Geometry check sheet. Reference: the model listing, model coordinates, mm. A direction names the side the tool comes from. Give positions to 0.01 mm unless a question says otherwise; leave off trailing zeros. Loops run counter-clockwise (first coordinate to the right, second up) from the corner with the lowest first, then second, coordinate; pieces in that order, holes last. Notation, with made-up numbers: (-33, 10) - (16, 10) arc R21 ccw to (16, 38) - close; hole circle Ø1 at (15.25, -1.5). An arc over 180 degrees is marked (long way). Write item = value, one per line. Start each with the question number.
Autodesk Inventor part; units mm, degrees
ref_plane "YZ Plane" through (0, 0, 0) normal (1, 0, 0) x (0, 1, 0)
ref_plane "XZ Plane" through (0, 0, 0) normal (0, 1, 0) x (-1, 0, 0)
ref_plane "XY Plane" through (0, 0, 0) normal (0, 0, 1) x (1, 0, 0)
sketch "Sketch1" plane through (0, 0, 0) normal (0, 0, 1) x (1, 0, 0)
  line L0 (0, 0) -> (114.3, 0)
  line L1 (114.3, 0) -> (114.3, 25.4)
  line L2 (114.3, 25.4) -> (0, 25.4)
  line L3 (0, 25.4) -> (0, 0)
  dimension "d0" = 114.3
  dimension "d1" = 25.4
extrude "Plate1" add sketch "Sketch1" along normal blind 3.048
sketch "Sketch2" plane through (114.3, 22.352, 3.048) normal (0, 1, 0) x (-1, 0, 0)
  line L0 (114.3, 0) -> (0, 0)
  line L1 (0, 0) -> (0, -25.4)
  line L2 (0, -25.4) -> (114.3, -25.4)
  line L3 (114.3, -25.4) -> (114.3, 0)
edge flange "Flange1" height 25.4 angle 90 thickness 3.048 bend radius 3.048 thickness toward (0, 1, 0) relief tear relief width 3.048 relief depth 1.524 edges at (57.15, 25.4, 0) wall of the first edge with corners at (0, 22.352, 3.048) (114.3, 22.352, 3.048) (114.3, 22.352, -22.352) (0, 22.352, -22.352)
bend "Bend1"
corner "Corner1"
hole "Hole1" at (101.6, 9.652, 0) direction (0, 0, 1) diameter 6.35 end through all
hole "Hole2" at (25.4, 9.652, 0) direction (0, 0, 1) diameter 6.35 end through all
equation "\"d20\" = Thickness"
equation "\"d29\" = Thickness"
equation "\"d3\" = BendReliefWidth"
equation "\"d4\" = BendReliefDepth"
equation "\"d5\" = MinimumRemnant"
equation "\"d6\" = BendRadius"
equation "\"d9\" = BendRadius"
equation "\"d10\" = CornerReliefSize"
equation "\"d11\" = GapSize"
equation "\"d12\" = JacobiRadiusSize"
equation "\"BendRadius\" = Thickness"
equation "\"BendReliefWidth\" = Thickness"
equation "\"BendReliefDepth\" = 0.5 * Thickness"
equation "\"CornerReliefSize\" = 4 * Thickness"
equation "\"MinimumRemnant\" = 2 * Thickness"
equation "\"TransitionRadius\" = BendRadius"
equation "\"JacobiRadiusSize\" = BendRadius"
equation "\"GapSize\" = Thickness"
equation "\"d2\" = BendRadius"
properties part number "Chain Tension - L Bracket"
1) Cross-section at D-D on z = -1.5. Enter the section's corners in (x, y).
2) Tool access check on faces 4 (the face through (56, 10, 0)), 5 (the face through (58, 25.4, -13)). Record the directions out of +Z, -Z, +X, -X, +Y, -Y that give a thin tool (end or side, any length) a straight path to the whole face; none if there is none.
3) Cross-section at B-B on y = 10.5. Enter the section's corners in (x, z), and give its area (3 significant figures).
4) Material ranges on line 1 along Z through (x, y) = (109, 4.5); line 2 along Y through (x, z) = (98.5, -18.75); line 3 along Y through (x, z) = (25.4, 1), recorded low to high.
5) Cross-section at C-C on z = -15.5. Enter the section's corners in (x, y).
6) Cross-section at A-A on x = 25.4. Enter the section's corners in (y, z), and give its area (3 significant figures).
7) Gauge pin test, flat ends, axial feed: P1, Ø1, axis at x = 66, y = 8, coming from the -Z side; P2, Ø4, axis at x = 24.5, z = -12.5, coming from the -Y side; P3, Ø4, axis at x = 74.5, y = 22, coming from the +Z side; P4, Ø1.5, axis at y = 11.5, z = -2.5, coming from the -X side. Record the tip position at first contact, or that the pin passes through.
8) Release check for a two-part mould opening along Y. For faces 1 (the face through (58, 22.352, -13)), 2 (the face through (56, 10, 3.048)), 3 (the face through (104.7, 8.96, 1.55)) record: pulls with the +Y half, pulls with the -Y half, needs draft (parallel to the pull), parting line crosses it, or undercut.
Checked values:
q1.outline = (0, 21.93) - (114.3, 21.93) - (114.3, 25.2) - (0, 25.2) - close
q2.face_4 = -Z, +X, -X, -Y
q2.face_5 = +Z, -Z, +X, -X, +Y
q3.outline = (0, 0) - (22.34, 0) - (22.34, 3.05) - (0, 3.05) - close; (28.46, 0) - (98.54, 0) - (98.54, 3.05) - (28.46, 3.05) - close; (104.66, 0) - (114.3, 0) - (114.3, 3.05) - (104.66, 3.05) - close
q3.area = 311 mm²
q4.line_1 = 0 to 3.05
q4.line_2 = 22.35 to 25.4
q4.line_3 = 0 to 6.48, 12.83 to 23.86
q5.outline = (0, 22.35) - (114.3, 22.35) - (114.3, 25.4) - (0, 25.4) - close
q6.outline = (0, 0) - (6.48, 0) - (6.48, 3.05) - (0, 3.05) - close; (12.83, 0) - (19.3, 0) arc R3.05 cw to (22.35, -3.05) - (22.35, -22.35) - (25.4, -22.35) - (25.4, -3.05) arc R6.1 ccw to (19.3, 3.05) - (12.83, 3.05) - close
q6.area = 120 mm²
q7.P1 = 0
q7.P2 = 22.35
q7.P3 = 3.01
q7.P4 = through
q8.face_1 = pulls with the -Y half
q8.face_2 = needs draft
q8.face_3 = undercut
